Here's how the part is built. I have some questions about the finished solid (model axes, mm). Coordinates: 2 decimals unless noted, no trailing zeros. Write each loop counter-clockwise with the first axis right and the second up, starting at its lowest first coordinate (ties: lowest second). Pieces come first, ordered by that corner, then holes. Notation, with made-up numbers: (63, 18.25) -> (112, 18.25) arc R30 ccw to (112, 52.25) -> close; hole circle Ø2 at (-25, -33). An arc over 180 degrees is marked (long way). Use a Markdown table: item, result. Add a question column.
```python
from build123d import *

# Parameters (mm, degrees)
SKETCH_1_W          = 40
SKETCH_1_H          = 40
EXTRUDE_1_DEPTH     = 5
SKETCH_2_R          = 1.5
CUT_EXTRUDE_1_DEPTH = 10
FILLET_1_R          = 5
CUT_EXTRUDE_3_DEPTH = 3


with BuildPart() as part:
    # 草图1 → 凸台-拉伸1 (new body)
    with BuildSketch(Plane(origin=(0, 0, 0), x_dir=(1, 0, 0), z_dir=(0, 1, 0))):
        Rectangle(SKETCH_1_W, SKETCH_1_H)
    extrude(amount=EXTRUDE_1_DEPTH)

    # 草图2 → 切除-拉伸1 (cut)
    with BuildSketch(Plane(origin=(0, 5, 0), x_dir=(1, 0, 0), z_dir=(0, 1, 0))):
        with Locations((-15, 15)):
            Circle(SKETCH_2_R)
        with Locations((15, 15)):
            Circle(SKETCH_2_R)
        with Locations((15, -15)):
            Circle(SKETCH_2_R)
        with Locations((-15, -15)):
            Circle(SKETCH_2_R)
    extrude(amount=-CUT_EXTRUDE_1_DEPTH, mode=Mode.SUBTRACT)

    # 圆角1
    fillet_1_edges = [part.edges().sort_by_distance(p)[0] for p in [
        (20, 2.5, 20),
        (-20, 2.5, 20),
        (-20, 2.5, -20),
        (20, 2.5, -20),
    ]]
    fillet(fillet_1_edges, radius=FILLET_1_R)

    # 草图4 → 切除-拉伸3 (cut)
    with BuildSketch(Plane.XZ):
        Polygon((12.25, 16.58771324), (15, 18.175426481), (17.75, 16.58771324), (17.75, 13.41228676), (15, 11.824573519), (12.25, 13.41228676), align=None)
        Polygon((-15, 18.175426481), (-17.75, 16.58771324), (-17.75, 13.41228676), (-15, 11.824573519), (-12.25, 13.41228676), (-12.25, 16.58771324), align=None)
        Polygon((12.25, -13.41228676), (12.25, -16.58771324), (15, -18.175426481), (17.75, -16.58771324), (17.75, -13.41228676), (15, -11.824573519), align=None)
        Polygon((-12.25, -16.58771324), (-15, -18.175426481), (-17.75, -16.58771324), (-17.75, -13.41228676), (-15, -11.824573519), (-12.25, -13.41228676), align=None)
    extrude(amount=-CUT_EXTRUDE_3_DEPTH, mode=Mode.SUBTRACT)


solid = part.part
```
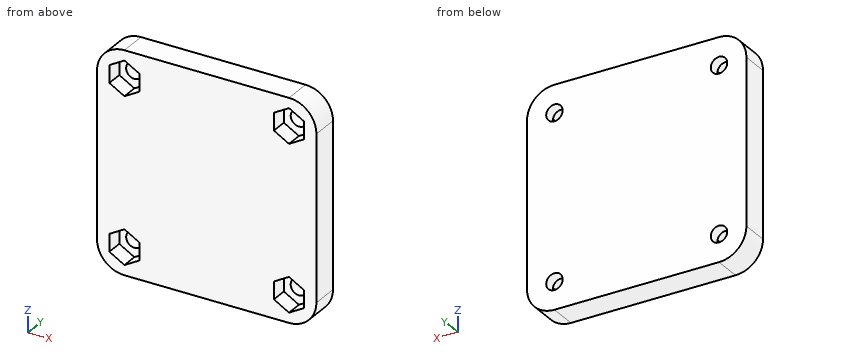
Q1. Please list where these lines run through material, in increasing order: line 1 (X direction, y = 3.75, z = 15); line 2 (Z direction, x = 15, y = 2.75).
Q2. Suppose I cut it at A-A, the plane y = 4.3. Write out the boundary of the cut face in (x, z).
Q3. Suppose I cut it at D-D, the plane y = 0.9. State how many separate pieces and enclosed holes the cut face has, and give its area (3 significant figures).
Q4. Will this pin go through, and if not, where does the flat tip stop? pin 1 (1.6 mm diameter, centred on x = 16, z = 13.5, fed in from -Y).
Q5. Suppose I cut it at B-B, the plane z = -14. Write out the boundary of the cut face in (x, y), and give its area (3 significant figures).
Q6. Suppose I cut it at C-C, the plane x = 15.5. Write out the boundary of the cut face in (y, z), and give its area (3 significant figures).
Answer key:
| question | item | result |
|---|---|---|
| 1 | line 1 | x = -20 to -16.5, -13.5 to 13.5, 16.5 to 20 |
| 1 | line 2 | z = -20 to -18.18, -11.82 to 11.82, 18.18 to 20 |
| 2 | outline | (-20, -15) arc R5 ccw to (-15, -20) -> (15, -20) arc R5 ccw to (20, -15) -> (20, 15) arc R5 ccw to (15, 20) -> (-15, 20) arc R5 ccw to (-20, 15) -> close; hole circle Ø3 at (-15, -15); hole circle Ø3 at (-15, 15); hole circle Ø3 at (15, -15); hole circle Ø3 at (15, 15) |
| 3 | separate pieces | 1 |
| 3 | enclosed holes | 4 |
| 3 | area | 1,470 mm^2 |
| 4 | pin 1 | stops at y = 3 |
| 5 | outline | (-20, 0) -> (-17.75, 0) -> (-17.75, 3) -> (-16.12, 3) -> (-16.12, 5) -> (-20, 5) -> close; (-13.88, 3) -> (-12.25, 3) -> (-12.25, 0) -> (12.25, 0) -> (12.25, 3) -> (13.88, 3) -> (13.88, 5) -> (-13.88, 5) -> close; (16.12, 3) -> (17.75, 3) -> (17.75, 0) -> (20, 0) -> (20, 5) -> (16.12, 5) -> close |
| 5 | area | 158 mm^2 |
| 6 | outline | (0, -19.97) -> (5, -19.97) -> (5, -16.41) -> (3, -16.41) -> (3, -17.89) -> (0, -17.89) -> close; (0, -12.11) -> (3, -12.11) -> (3, -13.59) -> (5, -13.59) -> (5, 13.59) -> (3, 13.59) -> (3, 12.11) -> (0, 12.11) -> close; (0, 17.89) -> (3, 17.89) -> (3, 16.41) -> (5, 16.41) -> (5, 19.97) -> (0, 19.97) -> close |
| 6 | area | 154 mm^2 |
